Design review of the part built by this model. Coordinates are the model's own, in mm. Face numbers are marked on the shaded views. A direction names the side the tool comes from. Coordinates: 2 decimals unless noted, no trailing zeros. Write each loop counter-clockwise with the first axis right and the second up, starting at its lowest first coordinate (ties: lowest second). Pieces come first, ordered by that corner, then holes. Notation, with made-up numbers: (59, 47) -> (111, 47) arc R23 ccw to (111, 81) -> close; hole circle Ø4 at (52.25, 1). An arc over 180 degrees is marked (long way). Answer in a Markdown table with one row per item. Add a question column.
Item 1: Take a section at A-A, the plane y = 15.5. Write out the cut boundary in (x, z).
Item 2: Draft analysis for pull direction X (two halves, no side actions). For the marked faces 1, 2 and 3, state which applies: released by +X, released by -X, zero draft, split by the parting line, or undercut.
Item 3: Clearance check with flat-ended pins moving along their axes: P1, Ø6, axis at x = -42, z = 13, coming from the -Y side; P2, Ø1.5, axis at x = -46, z = 10.5, coming from the +Y side; P3, Ø0.8, axis at x = 65, z = 9, coming from the -Y side. State where each tip first meets the part, or that it passes through.
Item 4: To check wall thickness, follow line 1 (X direction, y = 8, z = 7); line 2 (Y direction, x = -56.5, z = 5.5); line 3 (Y direction, x = 8.5, z = 4.75). State the ranges of each line that lie inside material, in increasing order.
Item 5: For the marked faces 4, 5 and 6, list the 3-axis set-ups (+Z, -Z, +X, -X, +Y, -Y) from which the entire face can be reached by the end or side of a thin tool; tool diameter is ignored.
Item 6: Take a section at C-C, the plane z = 8.25. Give the number of separate pieces and of enclosed holes in the cut face, and give its area (3 significant figures).
from build123d import *
from OCP.BRepFilletAPI import BRepFilletAPI_MakeChamfer

# Parameters (mm, degrees)
BOSS_EXTRUDE1_DEPTH = 15
BOSS_EXTRUDE2_DEPTH = 15
SKETCH6_W           = 115
SKETCH6_H           = 1.3
CUT_EXTRUDE2_DEPTH  = 10
CUT_EXTRUDE3_DEPTH  = 10
CUT_EXTRUDE4_DEPTH  = 10
BOSS_EXTRUDE3_DEPTH = 1
CUT_EXTRUDE5_REACH  = 117.913
SKETCH10_W          = 115
SKETCH10_H          = 5.7
SKETCH13_W          = 20.2
SKETCH13_H          = 23
CUT_EXTRUDE6_DEPTH  = 111.121977825
FILLET1_R           = 6
SKETCH14_W          = 6
SKETCH14_H          = 31
CUT_EXTRUDE7_DEPTH  = 4.5
FILLET2_R           = 3
SKETCH16_W          = 10
SKETCH16_H          = 2.5
CUT_EXTRUDE8_DEPTH  = 1.8
CHAMFER1_SIZE       = 0.5
CHAMFER1_SIZE_2     = 0.623907076
CHAMFER2_SIZE       = 1
CHAMFER3_SIZE       = 5
CHAMFER3_SIZE2      = 1.339745962
CUT_EXTRUDE12_REACH = 112.118
CHAMFER4_SIZE       = 0.2
CHAMFER4_SIZE_2     = 0.141421356
SKETCH25_W          = 6
SKETCH25_H          = 12
BOSS_EXTRUDE6_DEPTH = 15
FILLET4_START       = -1
FILLET4_DEPTH       = 16
FILLET4_2_DEPTH     = 15
CUT_EXTRUDE15_DEPTH = 15
CUT_EXTRUDE16_DEPTH = 10
CHAMFER5_SIZE       = 0.5
CHAMFER5_SIZE2      = 0.353553391
CHAMFER6_SIZE       = 0.65
SKETCH29_W          = 10
SKETCH29_H          = 0.8
CUT_EXTRUDE17_DEPTH = 3.1


with BuildPart() as part:
    # Sketch3 → Boss-Extrude1 (new body)
    with BuildSketch(Plane.XY):
        Polygon((0, 0), (0, 20.2), (-20.2, 20.2), (-20.2, -10.8), (-26.2, -10.8), (-26.2, 49.2), (-69.1, 49.2), (-69.1, 55.2), (5.9, 55.2), (65.9, 55.2), (65.9, 45.2), (6, 45.2), (6, 0), align=None)
    extrude(amount=BOSS_EXTRUDE1_DEPTH)

    # Sketch4 → Boss-Extrude2 (add)
    with BuildSketch(Plane.XY.offset(15)):
        with BuildLine():
            Line((-88.1, 30.2), (-94.1, 30.2))
            ThreePointArc((-94.1, 30.2), (-86.77766953, 47.87766953), (-69.1, 55.2))
            Line((-69.1, 55.2), (-69.1, 49.2))
            ThreePointArc((-69.1, 49.2), (-82.535028843, 43.635028843), (-88.1, 30.2))
        make_face()
    extrude(amount=-BOSS_EXTRUDE2_DEPTH)

    # Sketch6 → Cut-Extrude2 (cut)
    with BuildSketch(Plane.XY.offset(15)):
        with Locations((-11.6, 52.75)):
            Rectangle(SKETCH6_W, SKETCH6_H)
    extrude(amount=-CUT_EXTRUDE2_DEPTH, mode=Mode.SUBTRACT)

    # Sketch7 → Cut-Extrude3 (cut)
    with BuildSketch(Plane.XY.offset(15)):
        with BuildLine():
            Line((-92.3, 30.2), (-91, 30.2))
            ThreePointArc((-91, 30.2), (-84.585638508, 45.685638508), (-69.1, 52.1))
            Line((-69.1, 52.1), (-69.1, 53.4))
            ThreePointArc((-69.1, 53.4), (-85.504877324, 46.604877324), (-92.3, 30.2))
        make_face()
    extrude(amount=-CUT_EXTRUDE3_DEPTH, mode=Mode.SUBTRACT)

    # Sketch8 → Cut-Extrude4 (cut)
    with BuildSketch(Plane.XY.offset(15)):
        Polygon((45.9, 53.4), (65.9, 53.4), (65.9, 48.4), (45.9, 52.1), align=None)
    extrude(amount=-CUT_EXTRUDE4_DEPTH, mode=Mode.SUBTRACT)

    # Sketch9 → Boss-Extrude3 (add)
    with BuildSketch(Plane.XY.offset(15)):
        with BuildLine():
            Line((-69.1, 52.1), (45.9, 52.1))
            Line((45.9, 52.1), (45.9, 53.4))
            Line((45.9, 53.4), (-69.1, 53.4))
            ThreePointArc((-69.1, 53.4), (-85.504877324, 46.604877324), (-92.3, 30.2))
            Line((-92.3, 30.2), (-91, 30.2))
            ThreePointArc((-91, 30.2), (-84.585638508, 45.685638508), (-69.1, 52.1))
        make_face()
    extrude(amount=-BOSS_EXTRUDE3_DEPTH)

    # Cut-Extrude5: up to this face of the body (flat: up to its plane)
    cut_extrude5_end = Plane(part.part.faces().sort_by_distance((-11.6, 52.1, 9.5))[0])
    # Sketch10 → Cut-Extrude5 (cut, up to the picked face)
    with BuildSketch(Plane(origin=(0, 55.2, 0), x_dir=(-1, 0, 0), z_dir=(0, 1, 0)), mode=Mode.PRIVATE) as cut_extrude5_sk1:
        with Locations((11.6, 8.65)):
            Rectangle(SKETCH10_W, SKETCH10_H)
    cut_extrude5_tool1 = split(extrude(cut_extrude5_sk1.sketch, amount=-CUT_EXTRUDE5_REACH, mode=Mode.PRIVATE), bisect_by=cut_extrude5_end, keep=Keep.BOTH, mode=Mode.PRIVATE)
    add(cut_extrude5_tool1.solids().sort_by(Axis((-11.6, 55.2, 8.65), (0, -1, 0)))[0], mode=Mode.SUBTRACT)

    # Sketch13 → Cut-Extrude6 (cut, through all)
    with BuildSketch(Plane.XY.offset(15)):
        with Locations((-10.1, 37.7)):
            Rectangle(SKETCH13_W, SKETCH13_H)
    extrude(amount=-CUT_EXTRUDE6_DEPTH, mode=Mode.SUBTRACT)

    # Fillet1
    fillet1_edges = [part.edges().sort_by_distance(p)[0] for p in [
        (-20.2, 26.2, 7.5),
        (-20.2, 49.2, 7.5),
        (0, 49.2, 7.5),
        (0, 26.2, 7.5),
    ]]
    fillet(fillet1_edges, radius=FILLET1_R)

    # Sketch14 → Cut-Extrude7 (cut)
    with BuildSketch(Plane.XY.offset(15)):
        with Locations((-23.2, 4.7)):
            Rectangle(SKETCH14_W, SKETCH14_H)
    extrude(amount=-CUT_EXTRUDE7_DEPTH, mode=Mode.SUBTRACT)

    # Fillet2
    fillet2_edges = [part.edges().sort_by_distance(p)[0] for p in [
        (-26.2, 49.2, 7.5),
        (6, 45.2, 7.5),
        (-26.2, 20.2, 12.75),
        (6, 0, 7.5),
        (0, 0, 7.5),
        (-20.2, -10.8, 5.25),
        (-26.2, -10.8, 5.25),
    ]]
    fillet(fillet2_edges, radius=FILLET2_R - 0.0001)  # a hair under: the kernel refuses the full size

    # Sketch16 → Cut-Extrude8 (cut)
    with BuildSketch(Plane(origin=(0, 55.2, 0), x_dir=(-1, 0, 0), z_dir=(0, 1, 0))):
        with Locations((64.1, 12.75)):
            Rectangle(SKETCH16_W, SKETCH16_H)
    extrude(amount=-CUT_EXTRUDE8_DEPTH, mode=Mode.SUBTRACT)

    # Chamfer1
    # the kernel refuses this chamfer: 0.623907076, 0.5 mm, written as the material it takes off along each edge
    with BuildSketch(Plane(origin=(65.9, 55.2, -1.285841494), x_dir=(-1, 0, 0), z_dir=(0, 0, 1)), Plane(origin=(65.9, 45.2, -1.285841494), x_dir=(0, 1, 0), z_dir=(0, 0, 1))) as chamfer1_piece_1:
        Polygon((CHAMFER1_SIZE, 0), (0, CHAMFER1_SIZE), (0, 0), align=None)
    extrude(amount=17.571682988, mode=Mode.SUBTRACT)
    with BuildSketch(Plane(origin=(-88.1, 30.2, 16.303301327), x_dir=(-1, 0, 0), z_dir=(0, 0, -1))) as chamfer1_piece_2:
        with BuildLine():
            Line((CHAMFER1_SIZE, 0), (-0.006759226, 0.506759226))
            ThreePointArc((-0.006759226, 0.506759226), (-0.001786833, 0.26056951), (0, 0))
            Line((0, 0), (CHAMFER1_SIZE, 0))
        make_face()
    extrude(amount=17.606602654, mode=Mode.SUBTRACT)
    with BuildSketch(Plane(origin=(-94.1, 30.2, 16.285841494), x_dir=(1, 0, 0), z_dir=(0, 0, -1))) as chamfer1_piece_3:
        with BuildLine():
            Line((CHAMFER1_SIZE, 0), (0.004902903, -0.495097097))
            ThreePointArc((0.004902903, -0.495097097), (0.001296043, -0.254559377), (0, 0))
            Line((0, 0), (CHAMFER1_SIZE, 0))
        make_face()
    extrude(amount=17.571682988, mode=Mode.SUBTRACT)
    with BuildSketch(Plane(origin=(65.9, 53.4, 16.285841494), x_dir=(-1, 0, 0), z_dir=(0, 0, -1))) as chamfer1_piece_4:
        Polygon((CHAMFER1_SIZE, 0), (0, CHAMFER1_SIZE), (0, 0), align=None)
    extrude(amount=11.285841494, mode=Mode.SUBTRACT)
    with BuildSketch(Plane(origin=(65.9, 48.4, 16.611561789), x_dir=(-0.983314592491791, 0.18191319961097666, 0), z_dir=(0, 0, -1))) as chamfer1_piece_5:
        Polygon((CHAMFER1_SIZE, 0), (-CHAMFER1_SIZE_2 * 0.181913199708, -CHAMFER1_SIZE_2 * 0.983314593014), (0, 0), align=None)
    extrude(amount=11.611561789, mode=Mode.SUBTRACT)

    # Chamfer2
    chamfer2_edges = [part.edges().sort_by_distance(p)[0] for p in [
        (-10.1, 49.2, 15),
        (-10.1, 49.2, 0),
        (0, 37.7, 15),
        (0, 37.7, 0),
        (-10.1, 26.2, 15),
        (-10.1, 26.2, 0),
        (-20.2, 37.7, 15),
        (-20.2, 37.7, 0),
        (-1.757359313, 47.442640687, 15),
        (-1.757359313, 47.442640687, 0),
        (-1.757359313, 27.957359313, 15),
        (-1.757359313, 27.957359313, 0),
        (-18.442640687, 27.957359313, 15),
        (-18.442640687, 27.957359313, 0),
        (-18.442640687, 47.442640687, 15),
        (-18.442640687, 47.442640687, 0),
    ]]
    chamfer(chamfer2_edges, length=CHAMFER2_SIZE)

    # Chamfer3
    chamfer3_edges = [part.edges().sort_by_distance(p)[0] for p in [
        (45.9, 55.2, 8.65),
    ]]
    chamfer3_side = [part.faces().sort_by_distance(p)[0] for p in [
        (64.046661535, 55.2, 7.5),
    ]]
    chamfer(chamfer3_edges, length=CHAMFER3_SIZE, length2=CHAMFER3_SIZE2, reference=chamfer3_side[0])

    # Cut-Extrude12: up to this face of the body (flat: up to its plane)
    cut_extrude12_end = Plane(part.part.faces().sort_by_distance((-5.656799941, 54.307895333, 11.5))[0])
    # Sketch20 → Cut-Extrude12 (cut, up to the picked face)
    with BuildSketch(Plane.XY.offset(15), mode=Mode.PRIVATE) as cut_extrude12_sk1:
        Polygon((45.9, 52.1), (42.8, 55.2), (44.1, 55.2), (45.9, 53.4), align=None)
    cut_extrude12_tool1 = split(extrude(cut_extrude12_sk1.sketch, amount=-CUT_EXTRUDE12_REACH, mode=Mode.PRIVATE), bisect_by=cut_extrude12_end, keep=Keep.BOTH, mode=Mode.PRIVATE)
    add(cut_extrude12_tool1.solids().sort_by(Axis((44.646259, 53.946259, 15), (0, 0, -1)))[0], mode=Mode.SUBTRACT)

    # Chamfer4
    # the kernel refuses this chamfer: 0.2, 0.141421356 mm, written as the material it takes off along each edge
    with BuildSketch(Plane(origin=(44.6, 53.4, 10.985663402), x_dir=(-0.7071067811865653, 0.7071067811865298, 0), z_dir=(0, 0, 1))) as chamfer4_piece_1:
        Polygon((CHAMFER4_SIZE, 0), (CHAMFER4_SIZE_2 * 0.707106782373, CHAMFER4_SIZE_2 * 0.707106782373), (0, 0), align=None)
    extrude(amount=3.014336598, mode=Mode.SUBTRACT)
    with BuildSketch(Plane(origin=(44.1, 55.2, 15.514336598), x_dir=(1, 0, 0), z_dir=(0, 0, -1))) as chamfer4_piece_2:
        Polygon((CHAMFER4_SIZE_2 * 1.00000000168, 0), (CHAMFER4_SIZE * 0.707106781187, CHAMFER4_SIZE * 0.707106781186), (0, 0), align=None)
    extrude(amount=4.528673195, mode=Mode.SUBTRACT)

    # Sketch25 → Boss-Extrude6 (add)
    with BuildSketch(Plane.XY.offset(15)):
        with Locations((9, 26.1)):
            Rectangle(SKETCH25_W, SKETCH25_H)
    extrude(amount=-BOSS_EXTRUDE6_DEPTH)

    # Fillet4: read off the stored shape, not the designer's step
    # Fillet4 outline → Fillet4 (cut)
    with BuildSketch(Plane.XY.offset(FILLET4_START)):
        with BuildLine():
            ThreePointArc((9, 32.1), (11.121320344, 31.221320344), (12, 29.1))
            Line((12, 29.1), (12, 32.1))
            Line((12, 32.1), (9, 32.1))
        make_face()
        with BuildLine():
            ThreePointArc((12, 23.1), (11.121320344, 20.978679656), (9, 20.1))
            Line((9, 20.1), (12, 20.1))
            Line((12, 20.1), (12, 23.1))
        make_face()
    extrude(amount=FILLET4_DEPTH, mode=Mode.SUBTRACT)

    # Fillet4 2 outline → Fillet4 2 (add)
    with BuildSketch(Plane.XY):
        with BuildLine():
            Line((6, 32.1), (9, 32.1))
            ThreePointArc((9, 32.1), (6.878679656, 32.978679656), (6, 35.1))
            Line((6, 35.1), (6, 32.1))
        make_face()
        with BuildLine():
            ThreePointArc((6, 17.1), (6.878679656, 19.221320344), (9, 20.1))
            Line((9, 20.1), (6, 20.1))
            Line((6, 20.1), (6, 17.1))
        make_face()
    extrude(amount=FILLET4_2_DEPTH)

    # Sketch26 → Cut-Extrude15 (cut)
    with BuildSketch(Plane.XY.offset(15)):
        Polygon((12, 29.1), (10, 29.1), (7.402667467, 31.1), (6, 31.1), (6, 21.1), (8.459958458, 21.1), (10, 23.1), (12, 23.1), align=None)
    extrude(amount=-CUT_EXTRUDE15_DEPTH, mode=Mode.SUBTRACT)

    # Sketch27 → Cut-Extrude16 (cut)
    with BuildSketch(Plane.XY.offset(15)):
        Polygon((62.9, 53.4), (61.1, 55.2), (62.1, 55.2), (63.9, 53.4), align=None)
    extrude(amount=-CUT_EXTRUDE16_DEPTH, mode=Mode.SUBTRACT)

    # Chamfer5: one chamfer whose edges measure the first distance from different faces: ONE call of the kernel's chamfer builder (chamfer() names one face for all edges)
    chamfer5_edges_1 = [part.edges().sort_by_distance(p)[0] for p in [
        (62.9, 53.4, 10),
    ]]
    chamfer5_side_1 = [part.faces().sort_by_distance(p)[0] for p in [
        (62, 54.3, 10),
    ]]
    chamfer5_edges_2 = [part.edges().sort_by_distance(p)[0] for p in [
        (62.1, 55.2, 10),
    ]]
    chamfer5_side_2 = [part.faces().sort_by_distance(p)[0] for p in [
        (63, 54.3, 10),
    ]]
    chamfer5 = BRepFilletAPI_MakeChamfer(part.part.solid().wrapped)
    for e in chamfer5_edges_1:
        chamfer5.Add(CHAMFER5_SIZE, CHAMFER5_SIZE2, e.wrapped, chamfer5_side_1[0].wrapped)  # the first distance lies on this face
    for e in chamfer5_edges_2:
        chamfer5.Add(CHAMFER5_SIZE, CHAMFER5_SIZE2, e.wrapped, chamfer5_side_2[0].wrapped)  # the first distance lies on this face
    add(Compound.cast(chamfer5.Shape()), mode=Mode.REPLACE)

    # Chamfer6
    chamfer6_edges = [part.edges().sort_by_distance(p)[0] for p in [
        (-7.320710678, 53.4, 14),
        (-11.6, 52.1, 14),
        (-84.585638508, 45.685638508, 14),
        (-85.504877324, 46.604877324, 14),
    ]]
    chamfer(chamfer6_edges, length=CHAMFER6_SIZE - 0.0001)  # a hair under: the kernel refuses the full size

    # Sketch29 → Cut-Extrude17 (cut)
    with BuildSketch(Plane(origin=(0, 55.2, 0), x_dir=(-1, 0, 0), z_dir=(0, 1, 0))):
        with Locations((-40.9, 5.4)):
            Rectangle(SKETCH29_W, SKETCH29_H)
    extrude(amount=-CUT_EXTRUDE17_DEPTH, mode=Mode.SUBTRACT)


solid = part.part
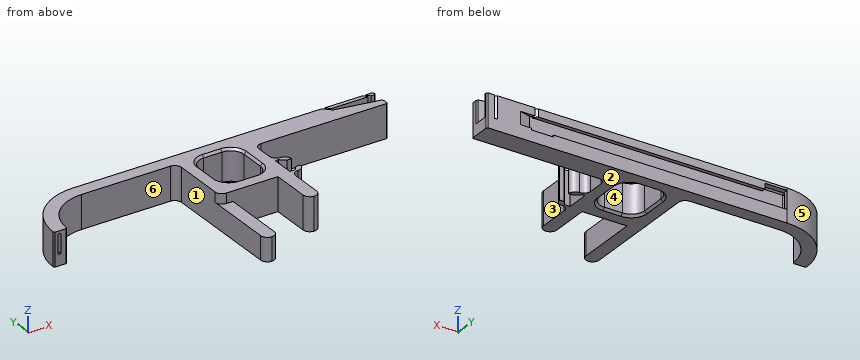
Answers:
| question | item | result |
|---|---|---|
| 1 | outline | (-26.2, 0) -> (-20.2, 0) -> (-20.2, 10.5) -> (-26.2, 10.5) -> close; (0, 0) -> (6, 0) -> (6, 15) -> (0, 15) -> close |
| 2 | face 1 | undercut |
| 2 | face 2 | zero draft |
| 2 | face 3 | released by +X |
| 3 | P1 | stops at y = 49.2 |
| 3 | P2 | stops at y = 52.1 |
| 3 | P3 | stops at y = 45.2 |
| 4 | line 1 | x = -26.2 to -20.2, 0 to 6 |
| 4 | line 2 | y = 49.2 to 52.1, 53.4 to 55.2 |
| 4 | line 3 | y = 20.06 to 21.15, 30.26 to 32.14, 45.16 to 55.2 |
| 5 | face 4 | +Z, -Z |
| 5 | face 5 | +Z, -Z, -X, +Y |
| 5 | face 6 | +Z, -Z, -Y |
| 6 | separate pieces | 4 |
| 6 | enclosed holes | 1 |
| 6 | area | 1,610 mm^2 |
